Could you check a few things on this model? Use its own coordinates, in mm. Round coordinates to 2 decimals unless told otherwise and drop trailing zeros. Write each loop counter-clockwise with the first axis right and the second up, starting at its lowest first coordinate (ties: lowest second). Pieces come first, ordered by that corner, then holes. Notation, with made-up numbers: (82.5, 55) -> (138.5, 55) arc R23 cw to (138.5, 72) -> close; hole circle Ø6 at (63, -1). An arc over 180 degrees is marked (long way). Answer as CSV lines item,"result". Start each with the question number.
Q1. If I drill on line 1 (Y direction, x = 18.5, z = 4.5) (3 decimals); line 2 (X direction, y = 32.5, z = 0.75); line 3 (X direction, y = 10.5, z = 1.05), over which ranges is the centre line in solid material (lowest first)? Write a range as [from, to].
Q2. Imagine slicing it at C-C on x = -18.75. Please give me the cut outline in (y, z).
Q3. Imagine slicing it at D-D on z = 2.8. Give the number of separate pieces and of enclosed holes in the cut face, and give its area (3 significant figures).
Q4. Imagine slicing it at A-A on y = -57. Please give me the cut outline in (x, z), and give its area (3 significant figures).
Q5. If we mould it in two halves opening along Y, with no side actions, what happens to faces 1 (the flat face through (16, -36.806, 3)), 2 (the flat face through (-1, -22, 5.08)), 3 (the flat face through (5.855, -55, 3)), 4 (the flat face through (-30.533, -5.139, 2.504))? For each: pulls with the +Y half, pulls with the -Y half, needs draft (parallel to the pull), parting line crosses it, or undercut.
Q6. Imagine slicing it at B-B on x = -30.5. Please give me the cut outline in (y, z).
Q7. Will these pins go through, and if not, where does the flat tip stop? pin 1 Ø1.5 at (y, z) = (-57, 1.5) entering from -X; pin 2 Ø1.5 at (y, z) = (-9, 1.5) entering from -X; pin 3 Ø1.5 at (y, z) = (14, 1.5) entering from +X.
from build123d import *

# Parameters (mm, degrees)
F0_R     = 1.65
F0_W     = 4.2823543772
F0_H     = 20.4163840114
F0_W_2   = 5
F0_H_2   = 27.6073180421
F1_DEPTH = 5.08


# Not quite as in the source:
# - a feature names something its author has since deleted; it is built from what else it names


with BuildPart() as f1:
    # F0 (on Top) → F1 (new body)
    with BuildSketch(Plane.XY):
        Polygon((21.25, 36.8060796608), (-21.25, 36.8060796608), (-42.5, 0), (-21.25, -36.8060796608), (-15.6452442706, -36.8060796608), (-9.6452442706, -36.8060796608), (-7.5036888061, -36.8060796608), (3.5473197586, -36.8060796608), (5.8547557294, -36.8060796608), (11.8547557294, -36.8060796608), (21.25, -36.8060796608), (42.5, 0), align=None)
        with Locations((-18.75, -32.4759526419)):
            Circle(F0_R, mode=Mode.SUBTRACT)
        with Locations((18.75, -32.4759526419)):
            Circle(F0_R, mode=Mode.SUBTRACT)
        with Locations((-37.5, 0)):
            Circle(F0_R, mode=Mode.SUBTRACT)
        with Locations((-18.75, 32.4759526419)):
            Circle(F0_R, mode=Mode.SUBTRACT)
        Polygon((-20.4496354018, 22.6038945413), (-16.75, 29.0118510268), (-2.0811383147, 29.0118510268), (2.2012160625, 29.0118510268), (16.75, 29.0118510268), (19.1722516141, 24.8163881624), (21.9975489559, 19.92282962), (33.5, 0), (27.7061208369, -10.0352930835), (25.125, -14.5059255134), (16.75, -29.0118510268), (2.497308068, -29.0118510268), (-2.502691932, -29.0118510268), (-16.75, -29.0118510268), (-25.125, -14.5059255134), (-27.6475357555, -10.1367654209), (-33.5, 0), (-23.1427541029, 17.9392761202), align=None, mode=Mode.SUBTRACT)
        with Locations((37.5, 0)):
            Circle(F0_R, mode=Mode.SUBTRACT)
        with Locations((18.75, 32.4759526419)):
            Circle(F0_R, mode=Mode.SUBTRACT)
        Polygon((2.2012160625, 8.5954670154), (-2.0811383147, 8.5954670154), (-9.4379286368, 8.5954670154), (-14.5152442706, 8.5954670154), (-14.5152442706, 6.9638797721), (-14.5152442706, 0), (-14.5152442706, -1.4045329846), (-8.1520013755, -1.4045329846), (-2.502691932, -1.4045329846), (2.497308068, -1.4045329846), (11.7475565604, -1.4045329846), (12.9847557294, -1.4045329846), (12.9847557294, 4.3822885496), (12.9847557294, 5.62991663), (12.9847557294, 8.5954670154), (8.9436992999, 8.5954670154), align=None)
        with Locations((-9.5152442706, 3.5954670154)):
            Circle(F0_R, mode=Mode.SUBTRACT)
        with Locations((7.9847557294, 3.5954670154)):
            Circle(F0_R, mode=Mode.SUBTRACT)
        Polygon((-9.6452442706, -36.8060796608), (-15.6452442706, -36.8060796608), (-15.6452442706, -73.3945329846), (-9.6452442706, -73.3945329846), (-9.6452442706, -69.4588214522), (-9.6452442706, -40.8093024077), align=None)
        Polygon((11.8547557294, -73.3945329846), (11.8547557294, -36.8060796608), (5.8547557294, -36.8060796608), (5.8547557294, -40.7417911932), (5.8547557294, -69.3913102377), (5.8547557294, -73.3945329846), align=None)
        Polygon((5.8547557294, -40.7417911932), (5.8547557294, -36.8060796608), (3.5473197586, -36.8060796608), (-1.9379455123, -50.3825876202), (0.0250296589, -55.1708695493), align=None)
        Polygon((-7.5036888061, -36.8060796608), (-9.6452442706, -36.8060796608), (-9.6452442706, -40.8093024077), (-3.8155182001, -55.0297430961), (-1.9379455123, -50.3825876202), align=None)
        Polygon((0.0250296589, -55.1708695493), (-1.9379455123, -50.3825876202), (-3.8155182001, -55.0297430961), (-1.8525430289, -59.8180250252), align=None)
        Polygon((-9.6452442706, -69.4588214522), (-9.6452442706, -73.3945329846), (-7.3378082997, -73.3945329846), (-1.8525430289, -59.8180250252), (-3.8155182001, -55.0297430961), align=None)
        Polygon((3.713200265, -73.3945329846), (5.8547557294, -73.3945329846), (5.8547557294, -69.3913102377), (0.0250296589, -55.1708695493), (-1.8525430289, -59.8180250252), align=None)
        Polygon((-9.6452442706, -73.3945329846), (-15.6452442706, -73.3945329846), (-15.6452442706, -83.3945329846), (11.8547557294, -83.3945329846), (11.8547557294, -73.3945329846), (5.8547557294, -73.3945329846), (3.713200265, -73.3945329846), (-7.3378082997, -73.3945329846), align=None)
        with Locations((-10.6452442706, -78.3945329846)):
            Circle(F0_R, mode=Mode.SUBTRACT)
        with Locations((6.8547557294, -78.3945329846)):
            Circle(F0_R, mode=Mode.SUBTRACT)
        Polygon((-9.4379286368, 8.5954670154), (-20.4496354018, 22.6038945413), (-23.1427541029, 17.9392761202), (-14.5152442706, 6.9638797721), (-14.5152442706, 8.5954670154), align=None)
        with Locations((0.0600388739, 18.8036590211)):
            Rectangle(F0_W, F0_H)
        Polygon((21.9975489559, 19.92282962), (19.1722516141, 24.8163881624), (8.9436992999, 8.5954670154), (12.9847557294, 8.5954670154), (12.9847557294, 5.62991663), align=None)
        Polygon((25.125, -14.5059255134), (27.7061208369, -10.0352930835), (12.9847557294, 4.3822885496), (12.9847557294, -1.4045329846), (11.7475565604, -1.4045329846), align=None)
        Polygon((-14.5152442706, 0), (-27.6475357555, -10.1367654209), (-25.125, -14.5059255134), (-8.1520013755, -1.4045329846), (-14.5152442706, -1.4045329846), align=None)
        with Locations((-0.002691932, -15.2081920057)):
            Rectangle(F0_W_2, F0_H_2)
    extrude(amount=F1_DEPTH)


solid = f1.part
Checks:
1,line 1,"[-36.806, -34.107], [-30.845, -25.981], [-8.018, -1.019], [14.376, 23.75], [25.981, 30.845], [34.107, 36.806]"
1,line 2,"[-23.74, -20.4], [-17.1, 17.1], [20.4, 23.74]"
1,line 3,"[-36.44, -27.44], [-17.29, -10.94], [-2.08, 2.2], [10.14, 16.06], [27.44, 36.44]"
2,outline,"(-36.81, 0) -> (-34.13, 0) -> (-34.13, 5.08) -> (-36.81, 5.08) -> close; (-30.83, 0) -> (-25.55, 0) -> (-25.55, 5.08) -> (-30.83, 5.08) -> close; (-9.59, 0) -> (-3.27, 0) -> (-3.27, 5.08) -> (-9.59, 5.08) -> close; (12.35, 0) -> (20.44, 0) -> (20.44, 5.08) -> (12.35, 5.08) -> close; (25.55, 0) -> (30.83, 0) -> (30.83, 5.08) -> (25.55, 5.08) -> close; (34.13, 0) -> (36.81, 0) -> (36.81, 5.08) -> (34.13, 5.08) -> close"
3,separate pieces,"1"
3,enclosed holes,"20"
3,area,"3,500 mm^2"
4,outline,"(-15.65, 0) -> (-9.65, 0) -> (-9.65, 5.08) -> (-15.65, 5.08) -> close; (-4.61, 0) -> (0.77, 0) -> (0.77, 5.08) -> (-4.61, 5.08) -> close; (5.85, 0) -> (11.85, 0) -> (11.85, 5.08) -> (5.85, 5.08) -> close"
4,area,"88.3 mm^2"
5,face 1,"pulls with the -Y half"
5,face 2,"needs draft"
5,face 3,"undercut"
5,face 4,"undercut"
6,outline,"(-20.78, 0) -> (-5.2, 0) -> (-5.2, 5.08) -> (-20.78, 5.08) -> close; (5.2, 0) -> (20.78, 0) -> (20.78, 5.08) -> (5.2, 5.08) -> close"
7,pin 1,"x = -15.65"
7,pin 2,"x = -37.74"
7,pin 3,"x = 34.85"
